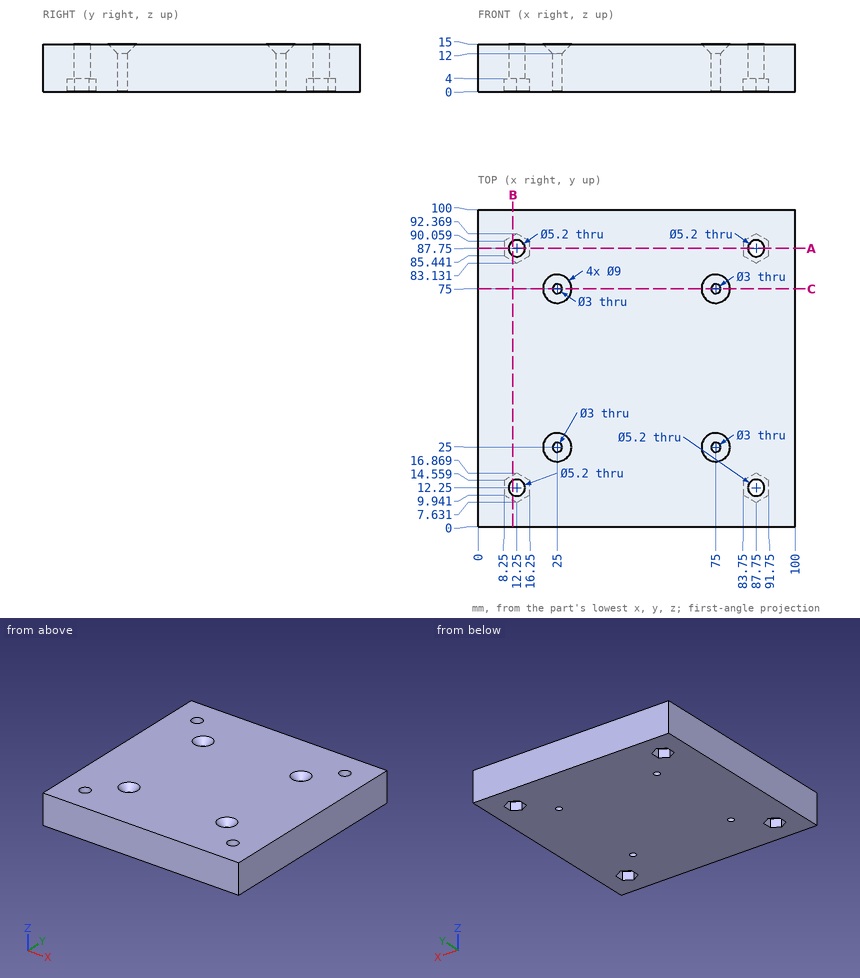
Here's the drawing with two shaded views (mm, measured from the low corner). I have some questions. Coordinates: 2 decimals unless noted, no trailing zeros. Loops run counter-clockwise (first coordinate to the right, second up) from the corner with the lowest first, then second, coordinate; pieces in that order, holes last. Notation, with made-up numbers: M 34.5,49.5 L 55.5,49.5 A38 cw 55.5,88.5 Z; hole C -13.75,-14.75 d2. An arc over 180 degrees is marked long. Put each result on its own line as item: value. Start each with the question number.
(1) Imagine slicing it at A-A on y = 87.75. List the corners of the cut face in (x, z) for me.
(2) Will these pins go through, and if not, where does the flat tip stop? pin 1 Ø4 at (x, y) = (75, 25) entering from +Z; pin 2 Ø3.5 at (x, y) = (25, 25) entering from +Z; pin 3 Ø4 at (x, y) = (89, 13) entering from -Z.
(3) Imagine slicing it at B-B on x = 11. List the corners of the cut face in (y, z) for me, and give its area (3 significant figures).
(4) I need wall thicknesses on probe 1 along Y at (x, z) = (87.75, 8.5); probe 2 along Y at (x, z) = (25, 4.25). Which ranges of each line are inside material? Lowest first, please.
(5) Imagine slicing it at C-C on y = 75. List the corners of the cut face in (x, z) for me, and give its area (3 significant figures).
Worked answers:
1. outline: M 0,0 L 8.25,0 L 8.25,4 L 9.65,4 L 9.65,15 L 0,15 Z; M 14.85,4 L 16.25,4 L 16.25,0 L 83.75,0 L 83.75,4 L 85.15,4 L 85.15,15 L 14.85,15 Z; M 90.35,4 L 91.75,4 L 91.75,0 L 100,0 L 100,15 L 90.35,15 Z
2. pin 1: stops at z = 12.5
2. pin 2: stops at z = 12.25
2. pin 3: stops at z = 4
3. outline: M 0,0 L 8.35,0 L 8.35,4 L 9.97,4 L 9.97,15 L 0,15 Z; M 14.53,4 L 16.15,4 L 16.15,0 L 83.85,0 L 83.85,4 L 85.47,4 L 85.47,15 L 14.53,15 Z; M 90.03,4 L 91.65,4 L 91.65,0 L 100,0 L 100,15 L 90.03,15 Z
3. area: 1,340 mm2
4. probe 1: y = 0 to 9.65, 14.85 to 85.15, 90.35 to 100
4. probe 2: y = 0 to 23.5, 26.5 to 73.5, 76.5 to 100
5. outline: M 0,0 L 23.5,0 L 23.5,12 L 20.5,15 L 0,15 Z; M 26.5,0 L 73.5,0 L 73.5,12 L 70.5,15 L 29.5,15 L 26.5,12 Z; M 76.5,0 L 100,0 L 100,15 L 79.5,15 L 76.5,12 Z
5. area: 1,390 mm2
